```python
from build123d import *

# Parameters (mm, degrees)
SKETCH2_R                                       = 51
BOSS_EXTRUDE1_DEPTH                             = 30.5
SKETCH3_R                                       = 46
CUT_EXTRUDE1_DEPTH                              = 20.5
M3_5X0_6_TAPPED_HOLE1_D                         = 2.9
F_6_0MM_DOWEL_HOLE1_D                           = 6
SKETCH10_R                                      = 38.5
SKETCH10_R_2                                    = 35.5
CUT_EXTRUDE2_DEPTH                              = 3
CBORE_FOR_M6_SOCKET_HEAD_CAP_SCREW1_D           = 6.6
CBORE_FOR_M6_SOCKET_HEAD_CAP_SCREW1_CBORE_D     = 11
CBORE_FOR_M6_SOCKET_HEAD_CAP_SCREW1_CBORE_DEPTH = 6


with BuildPart() as part:
    # Sketch2 → Boss-Extrude1 (new body)
    with BuildSketch(Plane.XY):
        Circle(SKETCH2_R)
    extrude(amount=BOSS_EXTRUDE1_DEPTH)

    # Sketch3 → Cut-Extrude1 (cut)
    with BuildSketch(Plane.XY.offset(30.5)):
        Circle(SKETCH3_R)
    extrude(amount=-CUT_EXTRUDE1_DEPTH, mode=Mode.SUBTRACT)

    # M3.5x0.6 Tapped Hole1 (through all)
    with Locations(Plane(origin=(0, 0, 0), x_dir=(-1, 0, 0), z_dir=(0, 0, -1))):
        with Locations((21, 36.373066959), (36.373066959, 21), (42, 0), (36.373066959, -21), (21, -36.373066959), (0, -42), (-21, -36.373066959), (-36.373066959, -21), (-42, 0), (-36.373066959, 21), (-21, 36.373066959), (0, 42)):
            Hole(M3_5X0_6_TAPPED_HOLE1_D / 2)

    # Ø6.0mm Dowel Hole1 (through all)
    with Locations(Plane(origin=(0, 0, 0), x_dir=(-1, 0, 0), z_dir=(0, 0, -1))):
        with Locations((-10.870399894, 40.568884704), (40.568884704, 10.870399894), (10.870399894, -40.568884704), (-40.568884704, -10.870399894)):
            Hole(F_6_0MM_DOWEL_HOLE1_D / 2)

    # Sketch10 → Cut-Extrude2 (cut)
    with BuildSketch(Plane.XY.offset(10)):
        Circle(SKETCH10_R)
        Circle(SKETCH10_R_2, mode=Mode.SUBTRACT)
    extrude(amount=-CUT_EXTRUDE2_DEPTH, mode=Mode.SUBTRACT)

    # CBORE for M6 Socket Head Cap Screw1 (through all)
    with Locations(Plane.XY.offset(10)):
        with Locations((0, 0)):
            CounterBoreHole(CBORE_FOR_M6_SOCKET_HEAD_CAP_SCREW1_D / 2, CBORE_FOR_M6_SOCKET_HEAD_CAP_SCREW1_CBORE_D / 2, CBORE_FOR_M6_SOCKET_HEAD_CAP_SCREW1_CBORE_DEPTH)


solid = part.part
```
Could you check a few things on this model? Use its own coordinates, in mm. A direction names the side the tool comes from. Round coordinates to 2 decimals unless told otherwise and drop trailing zeros. Loops run counter-clockwise (first coordinate to the right, second up) from the corner with the lowest first, then second, coordinate; pieces in that order, holes last.
Q1. On a 3-axis mill with a long thin cutter (end or side, diameter ignored), from which of +Z, -Z, +X, -X, +Y, -Y can I reach the whole of each face in a straight line? I mean faces 5 (the flat face through (11, -34, 7)), 6 (the cylindrical face through (2.43, 2.23, 1.97)). Say none if no direction works.
Q2. Thinking about a two-plate mould opening in Y: for faces 1 (the cylindrical face through (-1.19, -5.37, 7.04)), 2 (the cylindrical face through (-11.056, -49.787, 15.036)), 3 (the cylindrical face through (-30.55, -23.43, 8.52)), 4 (the flat face through (-8, 46, 30.5)), which applies, pulls with the +Y half, pulls with the -Y half, needs draft (parallel to the pull), parting line crosses it, or undercut?
Q3. Please list where these lines run through material, in increasing order: L1, parallel to Y at x = 1.5, z = 17; L2, parallel to X at y = 25.5, z = 7.5; L3, parallel to X at y = -12.5, z = 15.
Q4. I want a section at A-A (x = 0). Give the number of separate pieces and of enclosed holes in the cut face, and give its area (3 significant figures).
Q5. For P1, Ø5, axis at x = -10.87, y = -40.57, coming from the -Z side; P2, Ø23, axis at x = -14.5, y = 0.5, coming from the +Z side; P3, Ø1, axis at x = -32.5, z = 4.5, coming from the +Y side; P4, Ø6, axis at y = -13.5, z = 18, coming from the -X side, each with a flat end and sliding along its axis, tell me the tip position at first contact or that it passes through.
Q6. I want a section at B-B (y = -42). Write out the boundary of the cut face in (x, z), and give its area (3 significant figures).
Q7. I want a section at D-D (z = 13.5). Write out the boundary of the cut face in (x, y).
Q8. I want a section at C-C (x = -42). Write out the boundary of the cut face in (y, z).
Answer below:
1. face 5: +Z
1. face 6: +Z, -Z
2. face 1: undercut
2. face 2: parting line crosses it
2. face 3: undercut
2. face 4: needs draft
3. L1: y = -50.98 to -45.98, 45.98 to 50.98
3. L2: x = -44.17 to -28.84, -24.7 to 24.7, 28.84 to 44.17
3. L3: x = -49.44 to -44.27, 44.27 to 49.44
4. separate pieces: 4
4. enclosed holes: 0
4. area: 1,060 mm2
5. P1: passes through
5. P2: stops at z = 10
5. P3: stops at y = 39.71
5. P4: stops at x = -49.91
6. outline: (-28.93, 0) - (-13.51, 0) - (-13.51, 10) - (-18.76, 10) - (-18.76, 30.5) - (-28.93, 30.5) - close; (-8.23, 0) - (-1.45, 0) - (-1.45, 10) - (-8.23, 10) - close; (1.45, 0) - (28.93, 0) - (28.93, 30.5) - (18.76, 30.5) - (18.76, 10) - (1.45, 10) - close
6. area: 914 mm2
7. outline: circle Ø102 at (0, 0); hole circle Ø92 at (0, 0)
8. outline: (-28.93, 0) - (-1.45, 0) - (-1.45, 10) - (-18.76, 10) - (-18.76, 30.5) - (-28.93, 30.5) - close; (1.45, 0) - (8.23, 0) - (8.23, 10) - (1.45, 10) - close; (13.51, 0) - (28.93, 0) - (28.93, 30.5) - (18.76, 30.5) - (18.76, 10) - (13.51, 10) - close
